from build123d import *

# Parameters (mm, degrees)
F1_DEPTH = 25.4
F2_W     = 135.629368639
F2_H     = 58.648413825
F3_DEPTH = 12.7
F4_R     = 2.54
F5_SIZE  = 2.54


with BuildPart() as f1:
    # F0 (on Top) → F1 (new body)
    with BuildSketch(Plane.XY):
        with BuildLine():
            Line((-12.7, 0), (-148.329368639, 0))
            ThreePointArc((-148.329368639, 0), (-157.3096247601, -3.7197438789), (-161.029368639, -12.7))
            Line((-161.029368639, -12.7), (-161.029368639, -71.348413825))
            ThreePointArc((-161.029368639, -71.348413825), (-157.3096247601, -80.3286699461), (-148.329368639, -84.048413825))
            Line((-148.329368639, -84.048413825), (-12.7, -84.048413825))
            ThreePointArc((-12.7, -84.048413825), (-3.7197438789, -80.3286699461), (0, -71.348413825))
            Line((0, -71.348413825), (0, -12.7))
            ThreePointArc((0, -12.7), (-3.7197438789, -3.7197438789), (-12.7, 0))
        make_face()
    extrude(amount=F1_DEPTH)

    # F2 (on face) → F3 (cut)
    with BuildSketch(Plane.XY.offset(25.4)):
        with Locations((-80.5146843195, -42.0242069125)):
            Rectangle(F2_W, F2_H)
    extrude(amount=-F3_DEPTH, mode=Mode.SUBTRACT)

    # F4
    f4_edges = [f1.edges().sort_by_distance(p)[0] for p in [
        (-80.514684, -12.7, 25.4),
        (-80.514684, 0, 0),
        (-157.309625, -3.719744, 0),
        (-161.029369, -42.024207, 0),
        (-157.309625, -80.32867, 0),
        (-80.514684, -84.048414, 0),
        (-3.719744, -80.32867, 0),
        (0, -42.024207, 0),
        (-3.719744, -3.719744, 0),
    ]]
    fillet(f4_edges, radius=F4_R)

    # F5
    f5_edges = [f1.edges().sort_by_distance(p)[0] for p in [
        (-12.7, -42.024207, 12.7),
        (-80.514684, -12.7, 12.7),
        (-148.329369, -42.024207, 12.7),
        (-80.514684, -71.348414, 12.7),
        (-80.514684, -10.16, 25.4),
        (-148.329369, -42.024207, 25.4),
        (-80.514684, -71.348414, 25.4),
        (-12.7, -42.024207, 25.4),
    ]]
    chamfer(f5_edges, length=F5_SIZE)


solid = f1.part
Geometry: final body of the model. Coordinates: model frame, mm. A direction names the side the tool comes from. Round coordinates to 2 decimals unless told otherwise and drop trailing zeros. Loops run counter-clockwise (first coordinate to the right, second up) from the corner with the lowest first, then second, coordinate; pieces in that order, holes last. Notation, with made-up numbers: (-23, -8.5) - (36, -8.5) arc R20 cw to (36, 8.5) - close; hole circle Ø7 at (23, 12.5). An arc over 180 degrees is marked (long way). Write each question's results on one line, items separated by ' | '. Start each with the question number.
1) Cut plane B-B on x = -44. Return loops of the section in (y, z).
2) First-contact query: P1, Ø3, axis at x = -138, y = -16, coming from the +Z side; P2, Ø16, axis at x = -76, y = -42.5, coming from the +Z side. Flat tips, straight axial feed; report the tip coordinate or a pass-through.
3) Line query: probe 1 along X at (y, z) = (-58, 21.25); probe 2 along Y at (x, z) = (-19, 18.5); probe 3 along Z at (x, y) = (-135, -55.5). Output: solid intervals per line, ascending. Write a range as [from, to].
4) Access query for faces 1 (the face through (-82, -79, 25.4)), 2 (the face through (-12.7, -42, 19)). Directions: +Z, -Z, +X, -X, +Y, -Y. A direction counts if a zero-diameter tool reaches every point of the face in a straight line with its end or side. Return the directions, or none.
5) Cut plane A-A on z = 19.5. Return loops of the section in (x, y), then the cut area to 3 significant figures.
6) Cut plane C-C on y = -22. Return loops of the section in (x, z), then the cut area to 3 significant figures.
7) Mould query, pull axis X, two halves, no side actions, for faces 3 (the face through (-157.21, -3.62, 13.81)), 4 (the face through (-81, -84.048, 14)), 5 (the face through (-81, -71.348, 19)), 6 (the face through (-148.329, -42, 19)). Classes: released by +X, released by -X, zero draft, split by the parting line, or undercut.
Verdict:
1) outline: (-84.05, 2.54) arc R2.54 ccw to (-81.51, 0) - (-2.54, 0) arc R2.54 ccw to (0, 2.54) - (0, 25.4) - (-10.16, 25.4) arc R2.54 ccw to (-12.7, 22.86) - (-12.7, 15.24) - (-15.24, 12.7) - (-68.81, 12.7) - (-71.35, 15.24) - (-71.35, 22.86) - (-73.89, 25.4) - (-84.05, 25.4) - close
2) P1: stops at z = 13.44 | P2: stops at z = 12.7
3) probe 1: x = [-161.03, -148.33], [-12.7, 0] | probe 2: y = [-84.05, -71.35], [-12.7, 0] | probe 3: z = [0, 12.7]
4) face 1: +Z, +X, -X, +Y, -Y | face 2: +Z
5) outline: (-161.03, -71.35) arc R12.7 ccw to (-148.33, -84.05) - (-12.7, -84.05) arc R12.7 ccw to (0, -71.35) - (0, -12.7) arc R12.7 ccw to (-12.7, 0) - (-148.33, 0) arc R12.7 ccw to (-161.03, -12.7) - close; hole (-148.33, -71.35) - (-12.7, -71.35) - (-12.7, -12.7) - (-148.33, -12.7) - close | area: 5,440 mm2
6) outline: (-161.03, 2.54) arc R2.54 ccw to (-158.49, 0) - (-2.54, 0) arc R2.54 ccw to (0, 2.54) - (0, 25.4) - (-10.16, 25.4) - (-12.7, 22.86) - (-12.7, 15.24) - (-15.24, 12.7) - (-145.79, 12.7) - (-148.33, 15.24) - (-148.33, 22.86) - (-150.87, 25.4) - (-161.03, 25.4) - close | area: 2,360 mm2
7) face 3: released by -X | face 4: zero draft | face 5: undercut | face 6: undercut
